from build123d import *

# Parameters (mm, degrees)
F1_DEPTH = 17
F3_DEPTH = 17
F5_DEPTH = 17


# Not quite as in the source:
# - a pattern or mirror of a feature is missing from the dataset's text; its kind, count and spacing are read off the source's solid


with BuildPart() as f1:
    # F0 (on Right) → F1 (new body)
    with BuildSketch(Plane.YZ):
        Polygon((0, 24), (0, 0), (110, 0), (110, 24), (94.65, 24), (94.65, 17), (88.65, 17), (88.65, 13), (75.65, 13), (75.65, 17), (34.35, 17), (34.35, 13), (21.35, 13), (21.35, 17), (15.35, 17), (15.35, 24), align=None)
    extrude(amount=F1_DEPTH)

    # F2 (on face) → F3 (join, through all)
    with BuildSketch(Plane.YZ.offset(17)):
        Polygon((57.2362883389, 0), (55, 0), (55, -2), align=None)
        Polygon((55, 0), (52.7637116611, 0), (55, -2), align=None)
    extrude(amount=-F3_DEPTH)

    # F4 (on face) → F5 (join, through all)
    with BuildSketch(Plane.YZ.offset(17)):
        Polygon((0, 10.8757078871), (0, 13), (-2, 13), align=None)
        Polygon((-2, 13), (0, 13), (0, 15.1242921129), align=None)
    f5 = extrude(amount=-F5_DEPTH)

    # F5_copies: F5 across plane
    add(f5.mirror(Plane.ZX.offset(55)))


solid = f1.part
The listing builds one solid part. Answer for the finished solid, in the listing's coordinates (mm). A direction names the side the tool comes from. Give positions to 0.01 mm unless a question says otherwise; leave off trailing zeros. Write each loop counter-clockwise with the first axis right and the second up, starting at its lowest first coordinate (ties: lowest second). Pieces come first, ordered by that corner, then holes. Notation, with made-up numbers: (20.25, 86.25) -> (60.25, 86.25) arc R31 cw to (60.25, 122.25) -> close; hole circle Ø10 at (36, -28.5). An arc over 180 degrees is marked (long way). Use a Markdown table: item, result.
(1) Determine the mould class of faces 6 (the flat face through (8, 55, 17)), 7 (the flat face through (8, 18, 17)), 8 (the flat face through (8, 110, 5)), 9 (the flat face through (8, 83, 0)) for opening direction Y: released by +Y, released by -Y, zero draft, split by the parting line, or undercut.
Return value:
| item | result |
|---|---|
| face 6 | undercut |
| face 7 | undercut |
| face 8 | released by +Y |
| face 9 | zero draft |
(2) Section B-B, the plane x = 14.75 is taken. Determine the outline of the cut face in (y, z).
Return value:
| item | result |
|---|---|
| outline | (-2, 13) -> (0, 10.88) -> (0, 0) -> (52.76, 0) -> (55, -2) -> (57.24, 0) -> (110, 0) -> (110, 10.88) -> (112, 13) -> (110, 15.12) -> (110, 24) -> (94.65, 24) -> (94.65, 17) -> (88.65, 17) -> (88.65, 13) -> (75.65, 13) -> (75.65, 17) -> (34.35, 17) -> (34.35, 13) -> (21.35, 13) -> (21.35, 17) -> (15.35, 17) -> (15.35, 24) -> (0, 24) -> (0, 15.12) -> close |
(3) Section A-A, the plane z = 19.75 is taken. Determine the outline of the cut face in (x, y).
Return value:
| item | result |
|---|---|
| outline | (0, 0) -> (17, 0) -> (17, 15.35) -> (0, 15.35) -> close; (0, 94.65) -> (17, 94.65) -> (17, 110) -> (0, 110) -> close |
(4) Find the intervals of material crossed by probe 1 along Y at (x, z) = (9, 18.75); probe 2 along Z at (x, y) = (11.5, 73); probe 3 along Z at (x, y) = (10.75, 30), in increasing order. Write a range as from..to.
Return value:
| item | result |
|---|---|
| probe 1 | 0..15.35, 94.65..110 |
| probe 2 | 0..17 |
| probe 3 | 0..13 |
(5) Section D-D, the plane y = 69.5 is taken. Determine the outline of the cut face in (x, z), then the cut area to 3 significant figures.
Return value:
| item | result |
|---|---|
| outline | (0, 0) -> (17, 0) -> (17, 17) -> (0, 17) -> close |
| area | 289 mm2 |
(6) Flat-ended cylindrical pins translate along their axes: P1, Ø5, axis at x = 9.5, y = 93, coming from the +Z side; P2, Ø3, axis at x = 6.5, y = 54, coming from the -Z side; P3, Ø3, axis at x = 7.5, z = 15.5, coming from the -Y side; P4, Ø2, axis at x = 7, z = 19.5, coming from the -Y side. Find the tip coordinate at first contact, or state that the pin passes through.
Return value:
| item | result |
|---|---|
| P1 | z = 24 |
| P2 | z = -2 |
| P3 | y = -1.06 |
| P4 | y = 0 |
(7) Section C-C, the plane z = 14 is taken. Determine the outline of the cut face in (x, y).
Return value:
| item | result |
|---|---|
| outline | (0, -1.06) -> (17, -1.06) -> (17, 21.35) -> (0, 21.35) -> close; (0, 34.35) -> (17, 34.35) -> (17, 75.65) -> (0, 75.65) -> close; (0, 88.65) -> (17, 88.65) -> (17, 111.06) -> (0, 111.06) -> close |
(8) For faces 1 (the flat face through (8, 0, 6)), 2 (the flat face through (8.619, 56.102, -1.014)), 3 (the flat face through (8, 34.35, 15)), 4 (the flat face through (8, 110, 20)), 5 (the flat face through (8, 0, 20)), determine the directions among +Z, -Z, +X, -X, +Y, -Y from which every point of the face is accessible in a straight line to the end or side of a thin tool.
Return value:
| item | result |
|---|---|
| face 1 | -Z, +X, -X, -Y |
| face 2 | -Z, +X, -X, +Y |
| face 3 | +Z, +X, -X |
| face 4 | +Z, +X, -X, +Y |
| face 5 | +Z, +X, -X, -Y |
